Here's how the part is built. I have some questions about the finished solid (model axes, mm). Face numbers are marked on the shaded views. A direction names the side the tool comes from. Give positions to 0.01 mm unless a question says otherwise; leave off trailing zeros. Loops run counter-clockwise (first coordinate to the right, second up) from the corner with the lowest first, then second, coordinate; pieces in that order, holes last. Notation, with made-up numbers: (-3, 19) - (23, 19) arc R36 ccw to (23, 58) - close; hole circle Ø10 at (7, 44). An arc over 180 degrees is marked (long way). Return JSON: item names as keys, results as strings. Group by question number.
(1) If we section it at C-C (y = 19.05): Please give me the cut outline in (x, z).
(2) If we section it at D-D (x = 27): Please give me the cut outline in (y, z).
(3) If we section it at A-A (y = 12.7): Please give me the cut outline in (x, z).
(4) For P1, Ø12, axis at x = 13, y = 3.5, coming from the -Z side; P2, Ø4, axis at x = 41.5, z = -36, coming from the +Y side; P3, Ø7.5, axis at y = 6.5, z = -31, coming from the +X side, each with a flat end and sliding along its axis, tell me the tip position at first contact or that it passes through.
(5) If we section it at B-B (z = -32.5): Please give me the cut outline in (x, y), then the cut area to 3 significant figures.
(6) On a 3-axis mill with a long thin cutter (end or side, diameter ignored), from which of +Z, -Z, +X, -X, +Y, -Y can I reach the whole of each face in a straight line? I mean the marked faces 4, 5, 6, 7 and 8. Say none if no direction works.
(7) If we mould it in two halves opening along Y, with no side actions, what happens to the marked faces 1, 2 and 3? For each: released by +Y, released by -Y, zero draft, split by the parting line, or undercut.
(8) I need wall thicknesses on probe 1 along X at (y, z) = (19.5, -24.5); probe 2 along X at (y, z) = (4.5, -2); probe 3 along Z at (x, y) = (34.5, 12.7). Which ranges of each line are inside material? Lowest first, please. Write a range as [from, to].
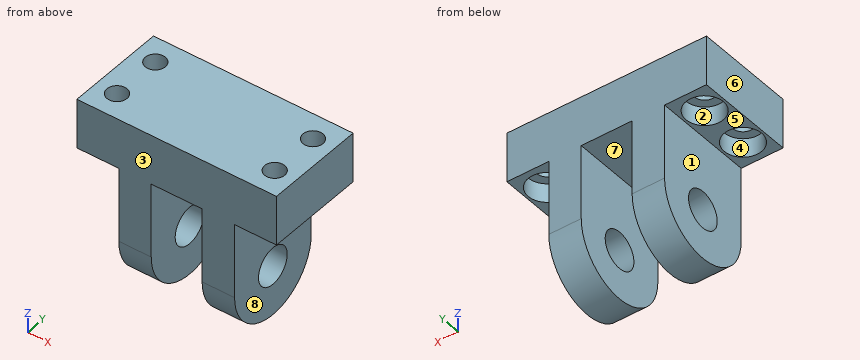
```python
from build123d import *

# Parameters (mm, degrees)
SKETCH1_R                                       = 4.7625
BOSS_EXTRUDE1_DEPTH                             = 50.8
CUT_EXTRUDE1_DEPTH                              = 26.4
CBORE_FOR_10_SOCKET_HEAD_CAP_SCREW1_D           = 5.1054
CBORE_FOR_10_SOCKET_HEAD_CAP_SCREW1_CBORE_D     = 9.525
CBORE_FOR_10_SOCKET_HEAD_CAP_SCREW1_CBORE_DEPTH = 4.826


with BuildPart() as part:
    # Sketch1 → Boss-Extrude1 (new body)
    with BuildSketch(Plane(origin=(0, 0, 0), x_dir=(0, 0, -1), z_dir=(1, 0, 0))):
        with BuildLine():
            Line((0, 0), (31.75, 0))
            ThreePointArc((31.75, 0), (44.45, 12.7), (31.75, 25.4))
            Line((31.75, 25.4), (0, 25.4))
            Line((0, 25.4), (0, 0))
        make_face()
        with Locations((31.75, 12.7)):
            Circle(SKETCH1_R, mode=Mode.SUBTRACT)
    extrude(amount=BOSS_EXTRUDE1_DEPTH)

    # Sketch2 → Cut-Extrude1 (cut, through all)
    with BuildSketch(Plane.XZ):
        Polygon((50.8, -12.7), (40.132, -12.7), (40.132, -44.45), (31.877, -44.45), (31.877, -12.7), (18.923, -12.7), (18.923, -44.45), (10.668, -44.45), (10.668, -12.7), (0, -12.7), (0, -50.8), (50.8, -50.8), align=None)
    extrude(amount=-CUT_EXTRUDE1_DEPTH, mode=Mode.SUBTRACT)

    # CBORE for #10 Socket Head Cap Screw1 (through all)
    with Locations(Plane(origin=(0, 0, -12.7), x_dir=(-1, 0, 0), z_dir=(0, 0, -1))):
        with Locations((-45.466, 6.35), (-45.466, 19.05), (-5.334, 19.05), (-5.334, 6.35)):
            CounterBoreHole(CBORE_FOR_10_SOCKET_HEAD_CAP_SCREW1_D / 2, CBORE_FOR_10_SOCKET_HEAD_CAP_SCREW1_CBORE_D / 2, CBORE_FOR_10_SOCKET_HEAD_CAP_SCREW1_CBORE_DEPTH)


solid = part.part
```
Values:
{
 "1": {"outline": "(0, -12.7) - (0.57, -12.7) - (0.57, -7.87) - (2.78, -7.87) - (2.78, 0) - (0, 0) - close; (7.89, -7.87) - (10.1, -7.87) - (10.1, -12.7) - (10.67, -12.7) - (10.67, -42.75) - (18.92, -42.75) - (18.92, -12.7) - (31.88, -12.7) - (31.88, -42.75) - (40.13, -42.75) - (40.13, -12.7) - (40.7, -12.7) - (40.7, -7.87) - (42.91, -7.87) - (42.91, 0) - (7.89, 0) - close; (48.02, -7.87) - (50.23, -7.87) - (50.23, -12.7) - (50.8, -12.7) - (50.8, 0) - (48.02, 0) - close"},
 "2": {"outline": "(0, -12.7) - (25.4, -12.7) - (25.4, 0) - (0, 0) - close"},
 "3": {"outline": "(0, -12.7) - (10.67, -12.7) - (10.67, -26.99) - (18.92, -26.99) - (18.92, -12.7) - (31.88, -12.7) - (31.88, -26.99) - (40.13, -26.99) - (40.13, -12.7) - (50.8, -12.7) - (50.8, 0) - (0, 0) - close; (10.67, -44.45) - (18.92, -44.45) - (18.92, -36.51) - (10.67, -36.51) - close; (31.88, -44.45) - (40.13, -44.45) - (40.13, -36.51) - (31.88, -36.51) - close"},
 "4": {"P1": "z = -44.04", "P2": "y = 25.09", "P3": "x = 40.13"},
 "5": {"outline": "(10.67, 0.02) - (18.92, 0.02) - (18.92, 8) - (10.67, 8) - close; (10.67, 17.4) - (18.92, 17.4) - (18.92, 25.38) - (10.67, 25.38) - close; (31.88, 0.02) - (40.13, 0.02) - (40.13, 8) - (31.88, 8) - close; (31.88, 17.4) - (40.13, 17.4) - (40.13, 25.38) - (31.88, 25.38) - close", "area": "263 mm2"},
 "6": {"face 4": "-Z", "face 5": "-Z, -X, +Y, -Y", "face 6": "+Z, -Z, -X, +Y, -Y", "face 7": "-Z, +Y, -Y", "face 8": "-Z, +X, +Y, -Y"},
 "7": {"face 1": "zero draft", "face 2": "undercut", "face 3": "released by -Y"},
 "8": {"probe 1": "[10.67, 18.92], [31.88, 40.13]", "probe 2": "[0, 3.58], [7.09, 43.71], [47.22, 50.8]", "probe 3": "[-44.45, -36.51], [-26.99, 0]"}
}
